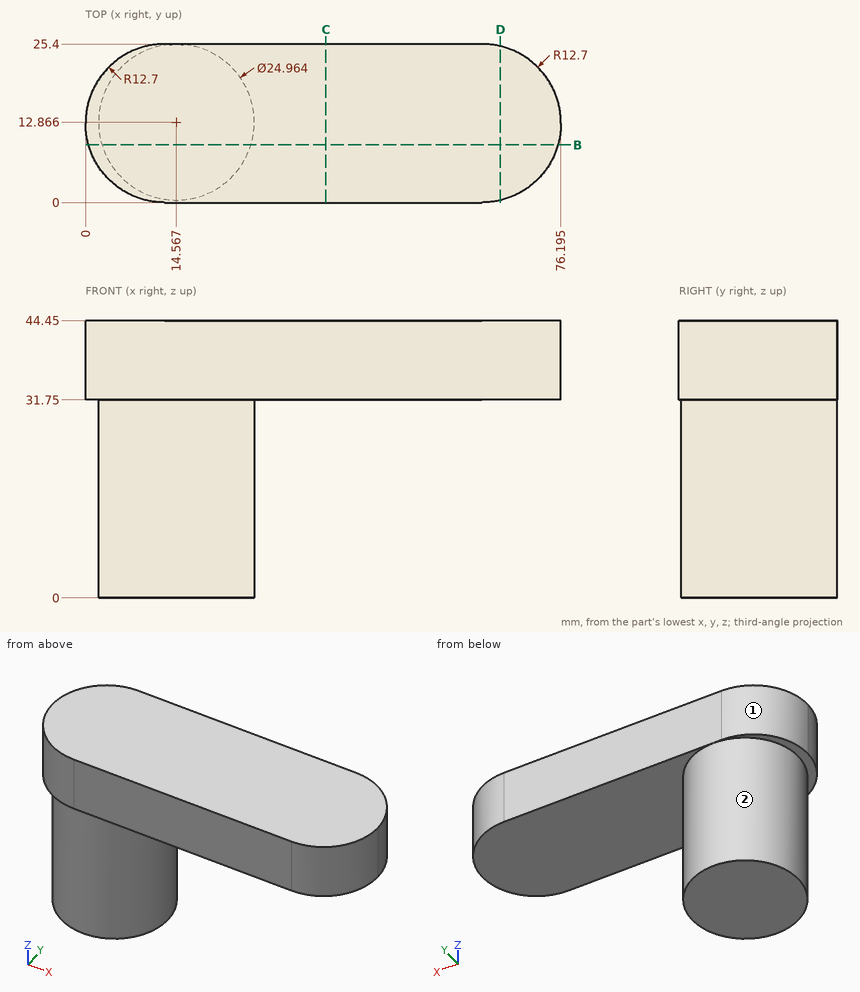
The figure shows three views and two pictorial views of one solid part (mm, origin at its lowest corner). Answer the questions. A direction names the side the tool comes from. Round coordinates to 2 decimals unless told otherwise and drop trailing zeros. Write each loop counter-clockwise with the first axis right and the second up, starting at its lowest first coordinate (ties: lowest second). Pieces come first, ordered by that corner, then holes. Notation, with made-up numbers: (50, 34.5) - (60, 34.5) arc R20 ccw to (60, 65.5) - close; hole circle Ø6 at (-24, 80.5). An arc over 180 degrees is marked (long way). Answer in a Markdown table with one row per item. Add a question column.
1. Find the intervals of material crossed by line 1 along Z through (x, y) = (4.5, 21); line 2 along X through (y, z) = (7.5, 35.5); line 3 along X through (y, z) = (9.5, 15), in increasing order. Write a range as from..to.
2. For the marked faces 1 and 2, determine the directions among +Z, -Z, +X, -X, +Y, -Y from which every point of the face is accessible in a straight line to the end or side of a thin tool.
3. A cutting plane is placed at B-B, the plane y = 9.25. Determine the outline of the cut face in (x, z).
4. A cutting plane is placed at C-C, the plane x = 38.5. Determine the outline of the cut face in (y, z), and give its area (3 significant figures).
5. A cutting plane is placed at D-D, the plane x = 66.5. Determine the outline of the cut face in (y, z).
6. Given pin 1 (2 mm diameter, centred on y = 10.5, z = 13.5, fed in from -X); pin 2 (1 mm diameter, centred on y = 10, z = 7.5, fed in from -X); pin 3 (1.5 mm diameter, centred on y = 6.5, z = 9.5, fed in from +X) (1 decimal); pin 4 (12 mm diameter, centred on x = 48, z = 22, fed in from -Y), each flat-ended and moving along its own axis, determine where each tip first touches the part or whether it passes through.
Worked out:
| question | item | result |
|---|---|---|
| 1 | line 1 | 31.75..44.45 |
| 1 | line 2 | 1.11..75.08 |
| 1 | line 3 | 2.55..26.59 |
| 2 | face 1 | +Z, -Z, -X, +Y |
| 2 | face 2 | -Z |
| 3 | outline | (0.48, 31.75) - (2.62, 31.75) - (2.62, 0) - (26.51, 0) - (26.51, 31.75) - (75.72, 31.75) - (75.72, 44.45) - (0.48, 44.45) - close |
| 4 | outline | (0, 31.75) - (25.4, 31.75) - (25.4, 44.45) - (0, 44.45) - close |
| 4 | area | 323 mm^2 |
| 5 | outline | (0.36, 31.75) - (25.04, 31.75) - (25.04, 44.45) - (0.36, 44.45) - close |
| 6 | pin 1 | x = 2.16 |
| 6 | pin 2 | x = 2.31 |
| 6 | pin 3 | x = 25.7 |
| 6 | pin 4 | through |
